```python
from build123d import *

# Parameters (mm, degrees)
F1_DEPTH = 1.75
F2_W     = 8.5
F2_H     = 2.5
F2_W_2   = 2.5
F2_H_2   = 12
F3_DEPTH = 1.75
F4_R     = 3
F5_DEPTH = 0.75


with BuildPart() as f1:
    # F0 (on Top) → F1 (new body)
    with BuildSketch(Plane.XY):
        with BuildLine():
            Line((-29.301108, -0.113589), (-29.301108, -16.636517))
            ThreePointArc((-29.301108, -16.636517), (-28.33456, -18.96997), (-26.001107, -19.936517))
            Line((-26.001107, -19.936517), (32.998893, -19.936517))
            ThreePointArc((32.998893, -19.936517), (35.332345, -18.96997), (36.298893, -16.636517))
            Line((36.298893, -16.636517), (36.298893, 7.363483))
            ThreePointArc((36.298893, 7.363483), (35.332345, 9.696936), (32.998893, 10.663484))
            Line((32.998893, 10.663484), (0.87364, 10.663484))
            ThreePointArc((0.87364, 10.663484), (2.222801, 13.64396), (-0.351107, 15.663484))
            Line((-0.351107, 15.663484), (-26.610989, 15.663484))
            ThreePointArc((-26.610989, 15.663484), (-28.481957, 14.890177), (-29.260977, 13.021579))
            Line((-29.260977, 13.021579), (-29.301108, -0.113589))
        make_face()
    extrude(amount=F1_DEPTH)

    # F2 (on face) → F3 (join, symmetric)
    with BuildSketch(Plane(origin=(0, 0, 0), x_dir=(1, 0, 0), z_dir=(0, 0, -1))):
        with Locations((24.548893, -11.913484)):
            Rectangle(F2_W, F2_H)
        with Locations((-30.550567, 5.936517)):
            Rectangle(F2_W_2, F2_H_2)
    extrude(amount=F3_DEPTH, both=True)

    # F4 (on face) → F5 (join)
    with BuildSketch(Plane.XY):
        with Locations((33.000201, -16.640954)):
            Circle(F4_R)
        with Locations((33.000201, 7.443574)):
            Circle(F4_R)
        with Locations((-26.091952, -16.551422)):
            Circle(F4_R)
        with Locations((-26.181484, 6.906373)):
            Circle(F4_R)
    extrude(amount=-F5_DEPTH)


solid = f1.part
```
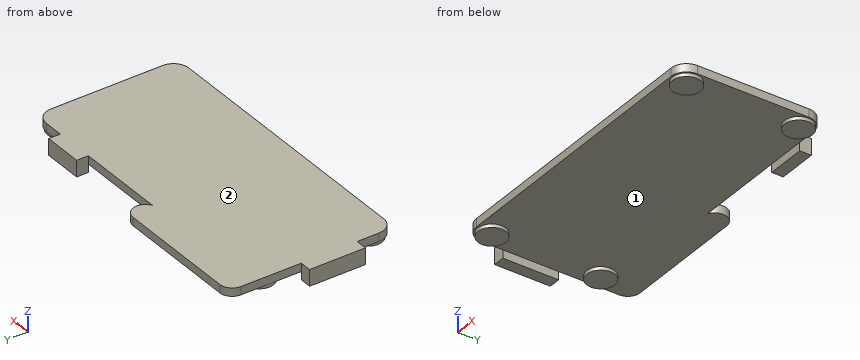
Design review of the part built by this model. Coordinates are the model's own, in mm. Face numbers are marked on the shaded views. Coordinates: 2 decimals unless noted, no trailing zeros. Loops run counter-clockwise (first coordinate to the right, second up) from the corner with the lowest first, then second, coordinate; pieces in that order, holes last. Notation, with made-up numbers: (81, -26.75) -> (90, -26.75) arc R36 cw to (90, 8.25) -> close; hole circle Ø8 at (51, 66). An arc over 180 degrees is marked (long way). Answer as a JSON object with one key per item and string values.
Q1. Take a section at A-A on y = 12. Give the boundary of the cut face in (x, z), plus the area to 3 significant figures.
Answer block:
{"outline": "(-29.26, 0) -> (2.1, 0) -> (2.1, 1.75) -> (-29.26, 1.75) -> close; (20.3, -1.75) -> (28.8, -1.75) -> (28.8, 1.75) -> (20.3, 1.75) -> close", "area": "84.6 mm^2"}
Q2. Take a section at B-B on x = 19.5. Give the boundary of the cut face in (y, z).
Answer block:
{"outline": "(-19.94, 0) -> (10.66, 0) -> (10.66, 1.75) -> (-19.94, 1.75) -> close"}
Q3. Take a section at C-C on y = -11. Give the boundary of the cut face in (x, z).
Answer block:
{"outline": "(-31.8, -1.75) -> (-29.3, -1.75) -> (-29.3, 0) -> (36.3, 0) -> (36.3, 1.75) -> (-31.8, 1.75) -> close"}
Q4. To check wall thickness, follow L1, parallel to Z at x = 29.5, y = 9; L2, parallel to X at y = -6.5, z = -1.4; L3, parallel to X at y = -14, z = 0.2. State the ranges of each line that lie inside material, in increasing order.
Answer block:
{"L1": "z = 0 to 1.75", "L2": "x = -31.8 to -29.3", "L3": "x = -29.3 to 36.3"}
Q5. Take a section at D-D on x = -3. Give the boundary of the cut face in (y, z), plus the area to 3 significant figures.
Answer block:
{"outline": "(-19.94, 0) -> (15.66, 0) -> (15.66, 1.75) -> (-19.94, 1.75) -> close", "area": "62.3 mm^2"}
Q6. The part is to be moulded in two halves that separate along X. For the marked faces 1 and 2, say which applies: +X half, -X half, draft (parallel to the pull), parting line (faces both ways), or undercut.
Answer block:
{"face 1": "undercut", "face 2": "draft"}
Q7. Clearance check with flat-ended pins moving along their axes: pin 1 Ø0.9 at (y, z) = (-14.5, 1.5) entering from -X; pin 2 Ø0.8 at (y, z) = (12.5, -0.5) entering from +X; pin 3 Ø5 at (x, y) = (-26, 7) entering from -Z. State where each tip first meets the part, or that it passes through.
Answer block:
{"pin 1": "stops at x = -29.3", "pin 2": "stops at x = 28.8", "pin 3": "stops at z = -0.75"}
